```python
from build123d import *

# Parameters (mm, degrees)
SKETCH1_W           = 22
SKETCH1_H           = 16
BOSS_EXTRUDE1_DEPTH = 20
CHAMFER1_SIZE       = 2
CHAMFER1_SIZE2      = 11.342563639
CUT_EXTRUDE1_DEPTH  = 20
FILLET1_R           = 10
SKETCH3_W           = 3.5
SKETCH3_H           = 10
BOSS_EXTRUDE2_DEPTH = 20
FILLET2_R           = 1
BOSS_EXTRUDE3_DEPTH = 3.5
SKETCH8_R           = 0.5
CUT_EXTRUDE2_DEPTH  = 3.5
SKETCH9_R           = 1.5
CUT_EXTRUDE3_DEPTH  = 6.5
SKETCH10_R          = 5
SKETCH10_R_2        = 0.5
BOSS_EXTRUDE4_DEPTH = 2.78


with BuildPart() as part:
    # Sketch1 → Boss-Extrude1 (new body)
    with BuildSketch(Plane.XY):
        with Locations((11, -8)):
            Rectangle(SKETCH1_W, SKETCH1_H)
    extrude(amount=BOSS_EXTRUDE1_DEPTH)

    # Chamfer1
    chamfer1_edges = [part.edges().sort_by_distance(p)[0] for p in [
        (0, 0, 10),
    ]]
    chamfer1_side = [part.faces().sort_by_distance(p)[0] for p in [
        (11, 0, 10),
    ]]
    chamfer(chamfer1_edges, length=CHAMFER1_SIZE, length2=CHAMFER1_SIZE2, reference=chamfer1_side[0])

    # Sketch2 → Cut-Extrude1 (cut)
    with BuildSketch(Plane.XY.offset(20)):
        Polygon((3.5, -16), (3.5, -14.5), (6.67, -14.5), (6.67, -12.5), (3.92, -12.5), (3.92, -10.5), (6.67, -10.5), (6.67, -6.5), (14.67, -6.5), (14.67, -10.5), (17.42, -10.5), (17.42, -12.5), (14.67, -12.5), (14.67, -14.5), (22, -14.5), (22, -16), align=None)
    extrude(amount=-CUT_EXTRUDE1_DEPTH, mode=Mode.SUBTRACT)

    # Fillet1
    fillet1_edges = [part.edges().sort_by_distance(p)[0] for p in [
        (0, -11.342563639, 10),
    ]]
    fillet(fillet1_edges, radius=FILLET1_R)

    # Sketch3 → Boss-Extrude2 (add)
    with BuildSketch(Plane.XZ.offset(16)):
        with Locations((1.75, 10)):
            Rectangle(SKETCH3_W, SKETCH3_H)
    extrude(amount=BOSS_EXTRUDE2_DEPTH)

    # Fillet2
    fillet2_edges = [part.edges().sort_by_distance(p)[0] for p in [
        (1.75, -16, 5),
        (1.75, -16, 15),
    ]]
    fillet(fillet2_edges, radius=FILLET2_R)

    # Sketch7 → Boss-Extrude3 (add)
    with BuildSketch(Plane.ZY):
        with BuildLine():
            Line((15, -36), (5, -36))
            ThreePointArc((5, -36), (10, -41), (15, -36))
        make_face()
    extrude(amount=-BOSS_EXTRUDE3_DEPTH)

    # Sketch8 → Cut-Extrude2 (cut)
    with BuildSketch(Plane.ZY):
        with Locations((10, -36)):
            Circle(SKETCH8_R)
    extrude(amount=-CUT_EXTRUDE2_DEPTH, mode=Mode.SUBTRACT)

    # Sketch9 → Cut-Extrude3 (cut)
    with BuildSketch(Plane.XZ.offset(6.5)):
        with Locations((10.67, 15)):
            Circle(SKETCH9_R)
        with Locations((10.67, 5)):
            Circle(SKETCH9_R)
    extrude(amount=-CUT_EXTRUDE3_DEPTH, mode=Mode.SUBTRACT)

    # Sketch10 → Boss-Extrude4 (add)
    with BuildSketch(Plane.ZY):
        with Locations((10, -36)):
            Circle(SKETCH10_R)
        with Locations((10, -36)):
            Circle(SKETCH10_R_2, mode=Mode.SUBTRACT)
    extrude(amount=BOSS_EXTRUDE4_DEPTH)


solid = part.part
```
Source: CAD feature listing. Evaluate the final solid. Frame: model axes, mm. A direction names the side the tool comes from. Coordinates: 2 decimals unless noted, no trailing zeros. Loops run counter-clockwise (first coordinate to the right, second up) from the corner with the lowest first, then second, coordinate; pieces in that order, holes last. Notation, with made-up numbers: M -6.5,13.25 L 2.5,13.25 A26 cw 2.5,42.25 Z; hole C 64,-40 d8. An arc over 180 degrees is marked long. Use a Markdown table: item, result. Add a question column.
Q1. First-contact query: pin 1 (6 mm diameter, centred on y = -20.5, z = 12.5, fed in from -X); pin 2 (8 mm diameter, centred on x = 4, z = 16.5, fed in from -Y); pin 3 (10 mm diameter, centred on y = -24, z = 6.5, fed in from +X); pin 4 (4 mm diameter, centred on y = -22.5, z = 2.5, fed in from +X). Flat tips, straight axial feed; report the tip coordinate or a pass-through.
Q2. Section query A-A, the plane z = 10. Return loops of the section in (x, y).
Q3. Section query D-D, the plane z = 17.5. Return loops of the section in (x, y).
Q4. Material intervals for L1, parallel to Z at x = 10.67, y = -3.75; L2, parallel to X at y = -13, z = 1.75; L3, parallel to Y at x = 4.25, z = 11.75, sorted ascending.
Q5. Section query B-B, the plane x = 10.67. Return loops of the section in (y, z), and give its area (3 significant figures).
Q6. Draft query along Y for faces 1 (the flat face through (11, -6.5, 10)), 2 (the flat face through (0, -21, 10)), 3 (the flat face through (16, -12.5, 10)). Return one class per face: pulls with the +Y half, pulls with the -Y half, needs draft (parallel to the pull), parting line crosses it, or undercut.
Q7. Access query for faces 4 (the flat face through (17.42, -11, 10)), 5 (the flat face through (18, -14.5, 10)), 6 (the flat face through (2, -26, 5)). Directions: +Z, -Z, +X, -X, +Y, -Y. A direction counts if a zero-diameter tool reaches every point of the face in a straight line with its end or side. Return the directions, or none.
Q8. Section query C-C, the plane y = -9. Return loops of the section in (x, z).
Result:
| question | item | result |
|---|---|---|
| 1 | pin 1 | stops at x = 0 |
| 1 | pin 2 | stops at y = -40.31 |
| 1 | pin 3 | stops at x = 3.5 |
| 1 | pin 4 | passes through |
| 2 | outline | M -2.78,-41 L 3.5,-41 L 3.5,-36.5 L -2.78,-36.5 Z; M -2.78,-35.5 L 3.5,-35.5 L 3.5,-14.5 L 6.67,-14.5 L 6.67,-12.5 L 3.92,-12.5 L 3.92,-10.5 L 6.67,-10.5 L 6.67,-6.5 L 14.67,-6.5 L 14.67,-10.5 L 17.42,-10.5 L 17.42,-12.5 L 14.67,-12.5 L 14.67,-14.5 L 22,-14.5 L 22,0 L 2,0 L 0.15,-10.48 A10 ccw 0,-12.22 L 0,-31 L -2.78,-31 Z |
| 3 | outline | M 0,-16 L 3.5,-16 L 3.5,-14.5 L 6.67,-14.5 L 6.67,-12.5 L 3.92,-12.5 L 3.92,-10.5 L 6.67,-10.5 L 6.67,-6.5 L 14.67,-6.5 L 14.67,-10.5 L 17.42,-10.5 L 17.42,-12.5 L 14.67,-12.5 L 14.67,-14.5 L 22,-14.5 L 22,0 L 2,0 L 0.15,-10.48 A10 ccw 0,-12.22 Z |
| 4 | L1 | z = 0 to 3.5, 6.5 to 13.5, 16.5 to 20 |
| 4 | L2 | x = 0 to 6.67, 14.67 to 22 |
| 4 | L3 | y = -14.5 to -12.5, -10.5 to 0 |
| 5 | outline | M -6.5,0 L 0,0 L 0,3.5 L -6.5,3.5 Z; M -6.5,6.5 L 0,6.5 L 0,13.5 L -6.5,13.5 Z; M -6.5,16.5 L 0,16.5 L 0,20 L -6.5,20 Z |
| 5 | area | 91.0 mm2 |
| 6 | face 1 | pulls with the -Y half |
| 6 | face 2 | needs draft |
| 6 | face 3 | undercut |
| 7 | face 4 | +Z, -Z |
| 7 | face 5 | +Z, -Z, +X, -Y |
| 7 | face 6 | -Z, +X, -X, -Y |
| 8 | outline | M 0.41,0 L 6.67,0 L 6.67,20 L 0.41,20 Z; M 14.67,0 L 22,0 L 22,20 L 14.67,20 Z |
